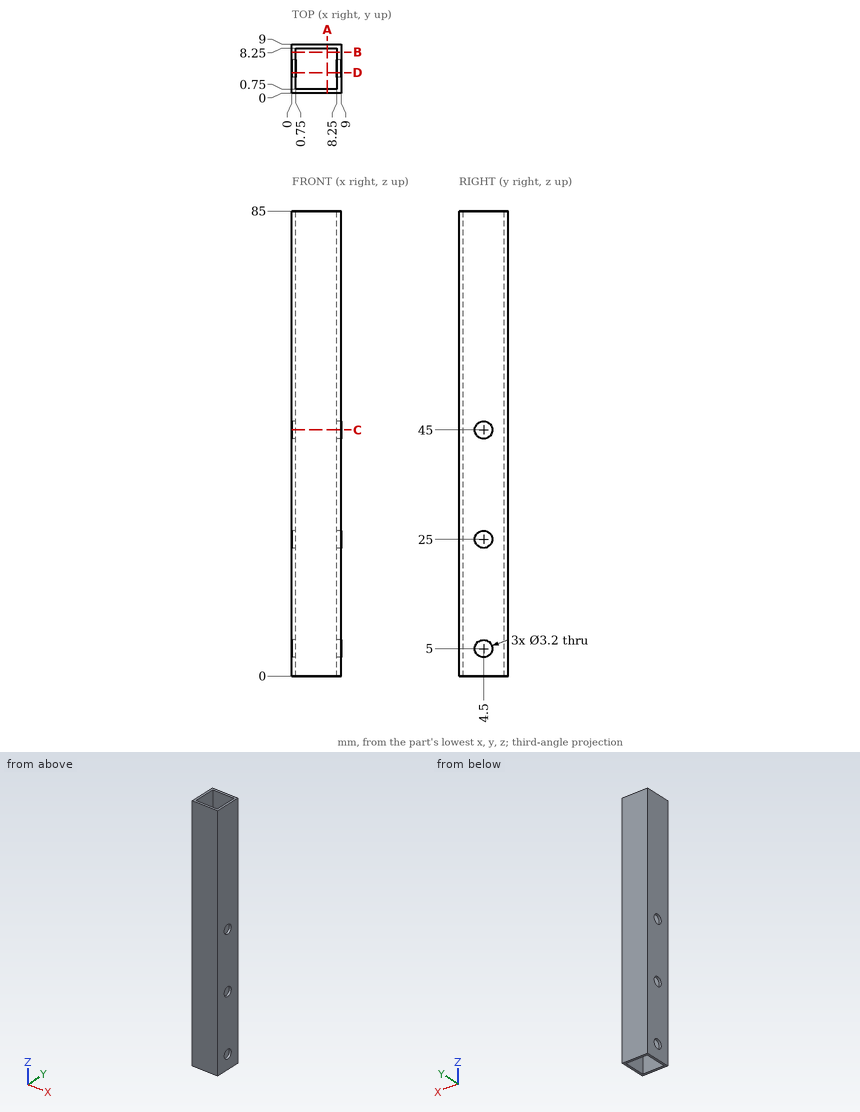
Geometry check sheet. Reference: drawing and pictorial views, mm from the part's lowest x, y, z. Coordinates: 2 decimals unless noted, no trailing zeros. Write each loop counter-clockwise with the first axis right and the second up, starting at its lowest first coordinate (ties: lowest second). Pieces come first, ordered by that corner, then holes.
Item 1: Cross-section at D-D on y = 3.75. Count the separate pieces of the cut face and the enclosed holes in it, then the cut area to 3 significant figures.
Numbers:
separate pieces: 8
enclosed holes: 0
area: 115 mm2
Item 2: Scan lines: probe 1 along Z at (x, y) = (8.55, 4.5); probe 2 along X at (y, z) = (7.25, 60); probe 3 along Y at (x, z) = (0.35, 45). Record each from-to range of solid material in increasing order.
Numbers:
probe 1: z = 0 to 3.4, 6.6 to 23.4, 26.6 to 43.4, 46.6 to 85
probe 2: x = 0 to 0.75, 8.25 to 9
probe 3: y = 0 to 2.9, 6.1 to 9
Item 3: Cross-section at C-C on z = 45. Record the boundary of the cut face in (x, y).
Numbers:
outline: (0, 0) - (9, 0) - (9, 2.9) - (8.25, 2.9) - (8.25, 0.75) - (0.75, 0.75) - (0.75, 2.9) - (0, 2.9) - close; (0, 6.1) - (0.75, 6.1) - (0.75, 8.25) - (8.25, 8.25) - (8.25, 6.1) - (9, 6.1) - (9, 9) - (0, 9) - close
Item 4: Cross-section at A-A on x = 6.5. Record the boundary of the cut face in (y, z).
Numbers:
outline: (0, 0) - (0.75, 0) - (0.75, 85) - (0, 85) - close; (8.25, 0) - (9, 0) - (9, 85) - (8.25, 85) - close
Item 5: Depth check by flat-ended pin: pin 1 Ø5 at (y, z) = (4.5, 5) entering from +X; pin 2 Ø1 at (x, y) = (2.5, 4) entering from +Z. Enter the tip coordinate at first touch or a pass-through.
Numbers:
pin 1: stops at x = 9
pin 2: passes through
